The listing builds one solid part. Answer for the finished solid, in the listing's coordinates (mm). A direction names the side the tool comes from. Coordinates: 2 decimals unless noted, no trailing zeros. Write each loop counter-clockwise with the first axis right and the second up, starting at its lowest first coordinate (ties: lowest second). Pieces come first, ordered by that corner, then holes.
(1) The part is cut by section D-D on z = 26. Determine the outline of the cut face in (x, y).
(2) Straight lines are drawn through the part: line 1 (X direction, y = 2.25, z = -19.5); line 2 (Z direction, x = -38.5, y = 7.75); line 3 (Z direction, x = -36, y = 11.5). For each, find the intervals that lie inside material, in ascending order.
(3) The part is cut by section C-C on z = 9.5. Determine the outline of the cut face in (x, y), plus the area to 3 significant figures.
(4) For a pull along Y with two mould halves and no side action, classify faces 4 (the flat face through (-32.998, 9, 40)), 5 (the flat face through (-30.533, 4.245, -24.969)), 6 (the flat face through (-43, 0, 7)) as +Y half, -Y half, draft (parallel to the pull), parting line (faces both ways), or undercut.
(5) The part is cut by section B-B on x = -30.5. Determine the outline of the cut face in (y, z), plus the area to 3 significant figures.
(6) Given P1, Ø4, axis at x = -37.5, y = 13.5, coming from the -Z side; P2, Ø3, axis at x = -38, y = 11.5, coming from the -Z side; P3, Ø10, axis at x = -43.5, z = 6, coming from the -Y side; P4, Ø7, axis at y = 5, z = -23.5, coming from the -X side, each flat-ended and moving along its own axis, determine where each tip first touches the part or whether it passes through.
(7) The part is cut by section A-A on x = -27. Determine the outline of the cut face in (y, z).
(8) Which of the six approach directions +Z, -Z, +X, -X, +Y, -Y give full straight-line access (tool end or side, diameter ignored) to faces 1 (the flat face through (-32.998, 9, -26)), 2 (the flat face through (-30.533, 4.136, 44.986)), 3 (the flat face through (-25, 9, 47.471))?
from build123d import *

# Parameters (mm, degrees)
BOSS_EXTRUDE1_DEPTH = 18
SKETCH2_R           = 1.75
CUT_EXTRUDE1_DEPTH  = 31.5
CUT_EXTRUDE2_DEPTH  = 1
CUT_EXTRUDE3_DEPTH  = 5


with BuildPart() as part:
    # Sketch1 → Boss-Extrude1 (new body)
    with BuildSketch(Plane(origin=(0, 0, 0), x_dir=(1, 0, 0), z_dir=(0, 1, 0))):
        with BuildLine():
            Line((-16.998275301, 32.528571429), (-32.998275301, 32.528571429))
            Line((-32.998275301, 32.528571429), (-32.998275301, 18.494895774))
            ThreePointArc((-32.998275301, 18.494895774), (-47.498275301, -7.471428571), (-32.998275301, -33.437752917))
            Line((-32.998275301, -33.437752917), (-32.998275301, -47.471428571))
            Line((-32.998275301, -47.471428571), (-16.998275301, -47.471428571))
            Line((-16.998275301, -47.471428571), (-16.998275301, -30.971428571))
            ThreePointArc((-16.998275301, -30.971428571), (-40.498275301, -7.471428571), (-16.998275301, 16.028571429))
            Line((-16.998275301, 16.028571429), (-16.998275301, 32.528571429))
        make_face()
    extrude(amount=BOSS_EXTRUDE1_DEPTH)

    # Sketch2 → Cut-Extrude1 (cut, through all)
    with BuildSketch(Plane(origin=(-16.998275301, 0, 0), x_dir=(0, 0, -1), z_dir=(1, 0, 0))):
        with Locations((-42.471428571, 5.25)):
            Circle(SKETCH2_R)
        with Locations((27.528571429, 5.25)):
            Circle(SKETCH2_R)
    extrude(amount=-CUT_EXTRUDE1_DEPTH, mode=Mode.SUBTRACT)

    # Sketch3 → Cut-Extrude2 (cut)
    with BuildSketch(Plane(origin=(-16.998275301, 0, 0), x_dir=(0, 0, -1), z_dir=(1, 0, 0))):
        Polygon((-41.871148795, 15.201025034), (-39.293157342, 15.201025034), (-39.293157342, 14.251238709), (-40.92136247, 14.251238709), (-40.92136247, 13.233610504), (-39.293157342, 13.233610504), (-39.293157342, 12.283824179), (-40.92136247, 12.283824179), (-40.92136247, 9.909358367), (-41.871148795, 9.909358367), align=None)
        with BuildLine():
            Line((-37.529268453, 13.912029308), (-38.479054777, 13.912029308))
            add(Edge.make_bspline(
                [(-38.479054777, 13.912029308), (-38.472348925, 13.959505738), (-38.459202545, 14.052580134), (-38.427745016, 14.187328674), (-38.390118416, 14.315146885), (-38.34314353, 14.435629995), (-38.288049629, 14.548992623), (-38.225396959, 14.655623774), (-38.154508221, 14.755065768), (-38.100171252, 14.814970019), (-38.073063525, 14.844855162)],
                knots=[0, 0, 0, 0, 0.000143778, 0.000281867, 0.000414671, 0.000543215, 0.000669322, 0.0007924, 0.000913902, 0.001034861, 0.001034861, 0.001034861, 0.001034861], degree=3))
            add(Edge.make_bspline(
                [(-38.073063525, 14.844855162), (-38.033964221, 14.884286443), (-37.956903602, 14.962001353), (-37.82812627, 15.061545568), (-37.693143844, 15.147694317), (-37.549249192, 15.215993668), (-37.398681424, 15.27127408), (-37.240243172, 15.308406058), (-37.074581872, 15.333043453), (-36.961538875, 15.335470322), (-36.903851118, 15.336708795)],
                knots=[0, 0, 0, 0, 0.000166428, 0.000328012, 0.000487119, 0.000645947, 0.000804887, 0.000967376, 0.001133328, 0.001306272, 0.001306272, 0.001306272, 0.001306272], degree=3))
            add(Edge.make_bspline(
                [(-36.903851118, 15.336708795), (-36.852563734, 15.335498), (-36.751743072, 15.333117822), (-36.603562067, 15.314011042), (-36.462283879, 15.280499879), (-36.326415158, 15.236684784), (-36.197954088, 15.177067025), (-36.07406541, 15.107863497), (-35.958210577, 15.022982493), (-35.850118512, 14.927075501), (-35.750815335, 14.8233427), (-35.664818348, 14.712460867), (-35.590885195, 14.597391911), (-35.529974057, 14.477179826), (-35.483141668, 14.3516212), (-35.450638602, 14.221441367), (-35.429364556, 14.08692758), (-35.427245105, 13.99550037), (-35.426170162, 13.949130336)],
                knots=[0, 0, 0, 0, 0.000153836, 0.00030241, 0.000447173, 0.000588968, 0.00072986, 0.000871333, 0.001014032, 0.001159723, 0.001304436, 0.001444171, 0.001580024, 0.001714184, 0.00184768, 0.001981114, 0.002116187, 0.002255197, 0.002255197, 0.002255197, 0.002255197], degree=3))
            add(Edge.make_bspline(
                [(-35.426170162, 13.949130336), (-35.428376009, 13.89170491), (-35.432718642, 13.778651902), (-35.468353097, 13.613190424), (-35.524130708, 13.454979724), (-35.604706892, 13.306233407), (-35.705447645, 13.167356277), (-35.829053175, 13.042991412), (-35.972002875, 12.931188942), (-36.079317119, 12.87110628), (-36.134269788, 12.840339604)],
                knots=[0, 0, 0, 0, 0.00017212, 0.000338852, 0.000505492, 0.00067385, 0.000844528, 0.001018431, 0.001198237, 0.00138694, 0.00138694, 0.00138694, 0.00138694], degree=3))
            add(Edge.make_bspline(
                [(-36.134269788, 12.840339604), (-36.096551119, 12.827955771), (-36.022435626, 12.803622094), (-35.917089364, 12.755697192), (-35.816917106, 12.703323219), (-35.723643783, 12.642478468), (-35.636341679, 12.575623232), (-35.555542998, 12.502186007), (-35.480764986, 12.422326922), (-35.413228364, 12.335606781), (-35.353286974, 12.243412505), (-35.299504756, 12.147873726), (-35.255238993, 12.047541582), (-35.21774038, 11.943561934), (-35.189191072, 11.835000267), (-35.169089807, 11.722277248), (-35.157470783, 11.605650007), (-35.155698684, 11.526635122), (-35.154802641, 11.486682085)],
                knots=[0, 0, 0, 0, 0.000119012, 0.000233852, 0.000346714, 0.000457856, 0.00056747, 0.000676282, 0.000785032, 0.000895296, 0.001005549, 0.001114686, 0.001223822, 0.001334132, 0.001445978, 0.001560132, 0.001677317, 0.001797176, 0.001797176, 0.001797176, 0.001797176], degree=3))
            add(Edge.make_bspline(
                [(-35.154802641, 11.486682085), (-35.156619041, 11.427967343), (-35.160200611, 11.31219383), (-35.182970562, 11.141671293), (-35.225364107, 10.979093204), (-35.281135164, 10.822588857), (-35.355527701, 10.674178666), (-35.443075211, 10.53045682), (-35.55068869, 10.396407552), (-35.670282595, 10.268486948), (-35.803098598, 10.152187262), (-35.947092752, 10.051360668), (-36.09909875, 9.964833512), (-36.260078289, 9.8945883), (-36.429975443, 9.840491454), (-36.608411526, 9.801387759), (-36.796136276, 9.777463472), (-36.924273105, 9.774955464), (-36.989713498, 9.773674607)],
                knots=[0, 0, 0, 0, 0.000176169, 0.00034737, 0.00051474, 0.000679386, 0.000844836, 0.001011921, 0.001183269, 0.001359492, 0.001536793, 0.001711778, 0.001885991, 0.002060677, 0.00223768, 0.002420033, 0.00260805, 0.002804296, 0.002804296, 0.002804296, 0.002804296], degree=3))
            add(Edge.make_bspline(
                [(-36.989713498, 9.773674607), (-37.051619054, 9.775025054), (-37.172667177, 9.777665676), (-37.349725391, 9.800521596), (-37.518002464, 9.837390049), (-37.677927841, 9.889359191), (-37.828882784, 9.956754287), (-37.972236212, 10.037006724), (-38.105127537, 10.134745277), (-38.229037432, 10.245557842), (-38.341217201, 10.369883248), (-38.441479496, 10.504841559), (-38.527613517, 10.650945966), (-38.599972501, 10.80757225), (-38.657990763, 10.974995181), (-38.703755398, 11.152874295), (-38.735722744, 11.341557113), (-38.745458467, 11.471374906), (-38.750422299, 11.537563496)],
                knots=[0, 0, 0, 0, 0.000185653, 0.000363021, 0.000534566, 0.000701839, 0.000866512, 0.001029812, 0.001193709, 0.001360353, 0.001527707, 0.001695195, 0.001863902, 0.002035591, 0.002211932, 0.002394731, 0.002586078, 0.002785121, 0.002785121, 0.002785121, 0.002785121], degree=3))
            Line((-38.750422299, 11.537563496), (-37.800635974, 11.537563496))
            add(Edge.make_bspline(
                [(-37.800635974, 11.537563496), (-37.794617277, 11.504283004), (-37.782894287, 11.439460519), (-37.760029312, 11.345611971), (-37.730233061, 11.258983964), (-37.695781181, 11.178806552), (-37.658567964, 11.104027033), (-37.613605499, 11.037407199), (-37.564188399, 10.977138049), (-37.492879164, 10.905489419), (-37.3909377, 10.831873443), (-37.253282951, 10.767897658), (-37.100155079, 10.730399988), (-36.993103425, 10.725825387), (-36.937772058, 10.723460932)],
                knots=[0, 0, 0, 0, 0.000101453, 0.000197607, 0.000289457, 0.000375893, 0.000459333, 0.000539595, 0.000616416, 0.00069287, 0.00084235, 0.000990791, 0.001145821, 0.001311674, 0.001311674, 0.001311674, 0.001311674], degree=3))
            add(Edge.make_bspline(
                [(-36.937772058, 10.723460932), (-36.90841128, 10.72396442), (-36.850900082, 10.724950642), (-36.766424697, 10.735881586), (-36.685949998, 10.753884861), (-36.609326097, 10.778350644), (-36.536065202, 10.809020032), (-36.467567036, 10.848566373), (-36.402435434, 10.89454464), (-36.341378437, 10.946236417), (-36.284960514, 11.002561951), (-36.238017483, 11.06493291), (-36.19511495, 11.128312952), (-36.163383928, 11.196848623), (-36.135580716, 11.266851971), (-36.11856373, 11.340863899), (-36.105714684, 11.417331835), (-36.104967949, 11.469663134), (-36.104588966, 11.49622235)],
                knots=[0, 0, 0, 0, 8.804e-05, 0.00017245, 0.000255004, 0.000335125, 0.000413489, 0.000492771, 0.000571884, 0.000652369, 0.000732575, 0.000810392, 0.000886249, 0.00096163, 0.001036443, 0.001111772, 0.00118898, 0.001268546, 0.001268546, 0.001268546, 0.001268546], degree=3))
            add(Edge.make_bspline(
                [(-36.104588966, 11.49622235), (-36.105595096, 11.525269377), (-36.10759807, 11.583095353), (-36.123962582, 11.667480206), (-36.149805605, 11.748651634), (-36.18570472, 11.82625017), (-36.233643988, 11.899989803), (-36.290211789, 11.971349973), (-36.35986473, 12.036616511), (-36.436283336, 12.101130505), (-36.524898897, 12.15736725), (-36.621395711, 12.209265504), (-36.728309865, 12.250560491), (-36.843031489, 12.287444563), (-36.967730649, 12.314384117), (-37.101633011, 12.333944858), (-37.244522568, 12.348504799), (-37.343018198, 12.350593662), (-37.393584692, 12.35166606)],
                knots=[0, 0, 0, 0, 8.7084e-05, 0.000173364, 0.000256838, 0.000342201, 0.000428949, 0.000520167, 0.000614623, 0.000714788, 0.000819753, 0.000928812, 0.001042981, 0.001163003, 0.001290052, 0.001425126, 0.001568892, 0.001720568, 0.001720568, 0.001720568, 0.001720568], degree=3))
            Line((-37.393584692, 12.35166606), (-37.393584692, 13.233610504))
            add(Edge.make_bspline(
                [(-37.393584692, 13.233610504), (-37.330626399, 13.238972234), (-37.212843901, 13.249002968), (-37.049355478, 13.272460189), (-36.911719301, 13.303814627), (-36.796627281, 13.34164206), (-36.701062242, 13.390222338), (-36.617577152, 13.44385282), (-36.545675843, 13.506136787), (-36.484909592, 13.57521694), (-36.436298482, 13.649402546), (-36.40189437, 13.727540541), (-36.379175692, 13.80721324), (-36.377023099, 13.861706965), (-36.375956487, 13.888708661)],
                knots=[0, 0, 0, 0, 0.000189544, 0.000354599, 0.000494992, 0.000612655, 0.000716948, 0.000815736, 0.000909673, 0.001001315, 0.001090992, 0.001174513, 0.001256793, 0.001337606, 0.001337606, 0.001337606, 0.001337606], degree=3))
            add(Edge.make_bspline(
                [(-36.375956487, 13.888708661), (-36.377796698, 13.923159894), (-36.3813884, 13.990401408), (-36.409283508, 14.086638178), (-36.457706253, 14.172425283), (-36.522632653, 14.247582201), (-36.601747728, 14.310358892), (-36.694484465, 14.355933699), (-36.798830471, 14.382710933), (-36.872243509, 14.38548683), (-36.910211295, 14.38692247)],
                knots=[0, 0, 0, 0, 0.000103264, 0.00020155, 0.000297405, 0.00039663, 0.000497784, 0.000598286, 0.000704469, 0.000818208, 0.000818208, 0.000818208, 0.000818208], degree=3))
            add(Edge.make_bspline(
                [(-36.910211295, 14.38692247), (-36.944624824, 14.385228566), (-37.012911806, 14.381867343), (-37.112767812, 14.356780059), (-37.20759775, 14.314548739), (-37.295437959, 14.256314238), (-37.375020447, 14.18637707), (-37.440334709, 14.103551012), (-37.494660015, 14.012798316), (-37.517687082, 13.945750658), (-37.529268453, 13.912029308)],
                knots=[0, 0, 0, 0, 0.000103172, 0.000204725, 0.000306758, 0.000413189, 0.000519795, 0.000623097, 0.000728547, 0.000835248, 0.000835248, 0.000835248, 0.000835248], degree=3))
        make_face()
    extrude(amount=-CUT_EXTRUDE2_DEPTH, mode=Mode.SUBTRACT)

    # Sketch4 → Cut-Extrude3 (cut)
    with BuildSketch(Plane.ZY.offset(32.998275301)):
        Polygon((-25.528765418, 2.783401278), (-24.392531269, 5.748583447), (-26.39233728, 8.215182169), (-29.528377439, 7.716598722), (-30.664611588, 4.751416553), (-28.664805577, 2.284817831), align=None)
        Polygon((44.362800811, 2.699305117), (45.626081257, 5.612628966), (43.734709018, 8.163323849), (40.580056332, 7.800694883), (39.316775886, 4.887371034), (41.208148125, 2.336676151), align=None)
    extrude(amount=-CUT_EXTRUDE3_DEPTH, mode=Mode.SUBTRACT)


solid = part.part
Model answer:
1. outline: (-41.23, 0) - (-31.45, 0) - (-31.45, 18) - (-41.23, 18) - close
2. line 1: x = -33 to -17
2. line 2: z = -14.16 to -2.01, 16.95 to 29.1
2. line 3: z = -16.39 to -6.36, 21.3 to 31.33
3. outline: (-47.43, 0) - (-40.41, 0) - (-40.41, 18) - (-47.43, 18) - close
3. area: 126 mm2
4. face 4: draft
4. face 5: undercut
4. face 6: -Y half
5. outline: (0, -32.53) - (18, -32.53) - (18, -11.76) - (0, -11.76) - close; (0, 26.71) - (18, 26.71) - (18, 47.47) - (0, 47.47) - close; hole (2.28, -28.66) - (4.75, -30.66) - (7.72, -29.53) - (8.22, -26.39) - (5.75, -24.39) - (2.78, -25.53) - close; hole (2.34, 41.21) - (4.89, 39.32) - (7.8, 40.58) - (8.16, 43.73) - (5.61, 45.63) - (2.7, 44.36) - close
5. area: 695 mm2
6. P1: stops at z = -16.78
6. P2: stops at z = -15.98
6. P3: stops at y = 0
6. P4: stops at x = -33
7. outline: (0, -32.53) - (18, -32.53) - (18, -13.79) - (0, -13.79) - close; (0, 28.74) - (18, 28.74) - (18, 47.47) - (0, 47.47) - close; hole circle Ø3.5 at (5.25, -27.53); hole circle Ø3.5 at (5.25, 42.47)
8. face 1: -Z, -X, +Y, -Y
8. face 2: -X
8. face 3: +Z, +X, -X, +Y, -Y
